Geometry check sheet. Reference: the model listing, model coordinates, mm. A direction names the side the tool comes from. Coordinates: 2 decimals unless noted, no trailing zeros. Write each loop counter-clockwise with the first axis right and the second up, starting at its lowest first coordinate (ties: lowest second). Pieces come first, ordered by that corner, then holes. Notation, with made-up numbers: (54.25, -38.5) -> (80.25, -38.5) arc R30 cw to (80.25, -13.5) -> close; hole circle Ø11 at (74, 77). An arc over 180 degrees is marked (long way). Answer in a Markdown table with one row per item. Add a question column.
1. Depth check by flat-ended pin: P1, Ø1, axis at y = 3.5, z = -1.5, coming from the -X side; P2, Ø1.5, axis at y = 3.5, z = -0.5, coming from the -X side; P3, Ø1, axis at x = -4, y = 2, coming from the -Z side. Enter the tip coordinate at first touch or a pass-through.
2. Cross-section at B-B on y = 3.75. Record the cut outline in (x, z), and give its area (3 significant figures).
3. Scan lines: L1, parallel to X at y = 0.1, z = -1.27; L2, parallel to Y at x = -22.25, z = -2.4; L3, parallel to X at y = 4, z = -0.25. Record each from-to range of solid material in increasing order. Write a range as from..to.
4. Mould release check, pull along X, two halves, no side actions. Record for faces 1 (the flat face through (-17.21, 3.13, -1.25)), 2 (the flat face through (-23.5, 0, -1.3)), 3 (the flat face through (-17.25, 3.41, -1.29)): pulls with the +X half, pulls with the -X half, needs draft (parallel to the pull), parting line crosses it, or undercut.
5. Cross-section at D-D on x = -10.25. Record the cut outline in (y, z).
6. Cross-section at C-C on x = -2.5. Record the cut outline in (y, z).
7. Set-up check for faces 4 (the flat face through (-8.32, 3.22, -1.25)), 5 (the flat face through (-24, 0.254, -2)), 6 (the flat face through (-2, 0, -1)), 7 (the flat face through (-2, 0.254, -1)): record each of +Z, -Z, +X, -X, +Y, -Y from which the full face is reachable in a straight line by a thin tool's end or side.
8. Cross-section at A-A on z = -1.27. Record the cut outline in (x, y), and give its area (3 significant figures).
```python
from build123d import *

# Parameters (mm, degrees)
SKETCH3_W                    = 2.54
SKETCH3_H                    = 0.254
F_69_0_0292_DIAMETER_HOLE1_D = 0.74168


with BuildPart() as part:
    # Sweep1: sweep along a path in Sketch2
    with BuildLine(Plane.XY) as sweep1_path:
        Line((0, 0), (-3.81, 0))
        Line((-3.81, 0), (-12.7, 6.35))
        Line((-12.7, 6.35), (-21.59, 0))
        Line((-21.59, 0), (-25.4, 0))
    # Sketch3 → Sweep1 (sweep)
    with BuildSketch(Plane(origin=(0, 0, 0), x_dir=(0, 0, -1), z_dir=(1, 0, 0))):
        with Locations((1.27, 0.127)):
            Rectangle(SKETCH3_W, SKETCH3_H)
    sweep(path=sweep1_path.line, transition=Transition.RIGHT)

    # #69 (0.0292) Diameter Hole1 (through all)
    with Locations(Plane(origin=(0, 0.254, 0), x_dir=(1, 0, 0), z_dir=(0, 1, 0))):
        with Locations((-24.0665, 1.27), (-1.3271754, 1.27)):
            Hole(F_69_0_0292_DIAMETER_HOLE1_D / 2)


solid = part.part
```
Results found:
| question | item | result |
|---|---|---|
| 1 | P1 | stops at x = -17.83 |
| 1 | P2 | stops at x = -18.18 |
| 1 | P3 | passes through |
| 2 | outline | (-16.78, -2.54) -> (-16.34, -2.54) -> (-16.34, 0) -> (-16.78, 0) -> close; (-9.06, -2.54) -> (-8.62, -2.54) -> (-8.62, 0) -> (-9.06, 0) -> close |
| 2 | area | 2.22 mm^2 |
| 3 | L1 | x = -25.4..-24.44, -23.7..-21.45, -3.95..-1.7, -0.96..0 |
| 3 | L2 | y = 0..0.25 |
| 3 | L3 | x = -16.43..-15.99, -9.41..-8.97 |
| 4 | face 1 | undercut |
| 4 | face 2 | needs draft |
| 4 | face 3 | pulls with the -X half |
| 5 | outline | (4.6, -2.54) -> (4.91, -2.54) -> (4.91, 0) -> (4.6, 0) -> close |
| 6 | outline | (0, -2.54) -> (0.25, -2.54) -> (0.25, 0) -> (0, 0) -> close |
| 7 | face 4 | +Z, -Z, -Y |
| 7 | face 5 | +Z, -Z, -X, +Y |
| 7 | face 6 | +Z, -Z, +X, -X, -Y |
| 7 | face 7 | +Z, -Z, +X, +Y |
| 8 | outline | (-25.4, 0) -> (-24.44, 0) -> (-24.44, 0.25) -> (-25.4, 0.25) -> close; (-23.7, 0) -> (-21.59, 0) -> (-12.7, 6.35) -> (-3.81, 0) -> (-1.7, 0) -> (-1.7, 0.25) -> (-3.73, 0.25) -> (-12.7, 6.66) -> (-21.67, 0.25) -> (-23.7, 0.25) -> close; (-0.96, 0) -> (0, 0) -> (0, 0.25) -> (-0.96, 0.25) -> close |
| 8 | area | 7.11 mm^2 |
